Read the model definition and answer for the solid it produces. Units are mm, in the model's axes. A direction names the side the tool comes from. Give positions to 0.01 mm unless a question says otherwise; leave off trailing zeros. Order: outer loops, then holes, each group sorted by start corner. A loop starts at its lowest first (then second) coordinate and runs counter-clockwise, first axis right, second up.
```python
from build123d import *

# Parameters (mm, degrees)
SKETCH_1_W          = 25
SKETCH_1_H          = 8
EXTRUDE_1_DEPTH     = 5.5
SKETCH_3_W          = 7
SKETCH_3_H          = 1.5
EXTRUDE_3_DEPTH     = 9
SKETCH_4_W          = 5
SKETCH_4_H          = 1.5
EXTRUDE_4_DEPTH     = 3.5
SKETCH_5_R          = 1.25
CUT_EXTRUDE_1_DEPTH = 2


with BuildPart() as part:
    # 草图1 → 凸台-拉伸1 (new body)
    with BuildSketch(Plane(origin=(0, 0, 0), x_dir=(1, 0, 0), z_dir=(0, 1, 0))):
        Rectangle(SKETCH_1_W, SKETCH_1_H)
    extrude(amount=EXTRUDE_1_DEPTH)

    # 草图3 → 凸台-拉伸3 (add)
    with BuildSketch(Plane.XY.offset(4)):
        with Locations((-6, 2.75)):
            Rectangle(SKETCH_3_W, SKETCH_3_H)
        with Locations((6, 2.75)):
            Rectangle(SKETCH_3_W, SKETCH_3_H)
    extrude(amount=EXTRUDE_3_DEPTH)

    # 草图4 → 凸台-拉伸4 (add)
    with BuildSketch(Plane(origin=(0, 0, -4), x_dir=(-1, 0, 0), z_dir=(0, 0, -1))):
        with Locations((-6, 2.75)):
            Rectangle(SKETCH_4_W, SKETCH_4_H)
        with Locations((6, 2.75)):
            Rectangle(SKETCH_4_W, SKETCH_4_H)
    extrude(amount=EXTRUDE_4_DEPTH)

    # 草图5 → 切除-拉伸1 (cut)
    with BuildSketch(Plane(origin=(0, 5.5, 0), x_dir=(1, 0, 0), z_dir=(0, 1, 0))):
        with Locations(Location((-10.25, 0, 0), (0, 0, 270))):
            Circle(SKETCH_5_R)
        with Locations(Location((10.25, 0, 0), (0, 0, 90))):
            Circle(SKETCH_5_R)
    extrude(amount=-CUT_EXTRUDE_1_DEPTH, mode=Mode.SUBTRACT)


solid = part.part
```
1) Consider L1, parallel to X at y = 4.35, z = 0; L2, parallel to Z at x = 10.25, y = 4.5; L3, parallel to X at y = 2.6, z = 12.25. Determine where each line is inside the solid, lowest interval first.
Final values:
L1: x = -12.5 to -11.5, -9 to 9, 11.5 to 12.5
L2: z = -4 to -1.25, 1.25 to 4
L3: x = -9.5 to -2.5, 2.5 to 9.5
2) The part is cut by section C-C on x = -10.25. Determine the outline of the cut face in (y, z), and give its area (3 significant figures).
Final values:
outline: (0, -4) - (5.5, -4) - (5.5, -1.25) - (3.5, -1.25) - (3.5, 1.25) - (5.5, 1.25) - (5.5, 4) - (0, 4) - close
area: 39.0 mm2
3) Given pin 1 (1.6 mm diameter, centred on y = 3, z = -6, fed in from +X); pin 2 (2 mm diameter, centred on x = -9.5, y = 4, fed in from -Z); pin 3 (0.8 mm diameter, centred on y = 2.5, z = 9.5, fed in from +X), each flat-ended and moving along its own axis, determine where each tip first touches the part or whether it passes through.
Final values:
pin 1: stops at x = 8.5
pin 2: stops at z = -4
pin 3: stops at x = 9.5
4) The part is cut by section D-D on z = 0. Determine the outline of the cut face in (x, y).
Final values:
outline: (-12.5, 0) - (12.5, 0) - (12.5, 5.5) - (11.5, 5.5) - (11.5, 3.5) - (9, 3.5) - (9, 5.5) - (-9, 5.5) - (-9, 3.5) - (-11.5, 3.5) - (-11.5, 5.5) - (-12.5, 5.5) - close
5) The part is cut by section B-B on y = 4.2. Determine the outline of the cut face in (x, z), and give its area (3 significant figures).
Final values:
outline: (-12.5, -4) - (12.5, -4) - (12.5, 4) - (-12.5, 4) - close; hole circle Ø2.5 at (-10.25, 0); hole circle Ø2.5 at (10.25, 0)
area: 190 mm2
6) A tool of negligible diameter and unlimited length cuts with its end or side. For faces 1 (the face through (-6, 3.5, 8)), 2 (the face through (-3.5, 3, -6)), 3 (the face through (10, 3.5, 0)), 4 (the face through (6, 2, -6)), from which of +Z, -Z, +X, -X, +Y, -Y can it reach the whole face along a straight path? Write none if from no direction.
Final values:
face 1: +Z, +X, -X, +Y
face 2: -Z, +Y, -Y
face 3: +Y
face 4: -Z, +X, -X, -Y
7) For a pull along X with two mould halves and no side action, classify faces 5 (the face through (0, 5.5, 0)), 6 (the face through (3.5, 3, -6)), 7 (the face through (8.5, 3, -6)) as released by +X, released by -X, zero draft, split by the parting line, or undercut.
Final values:
face 5: zero draft
face 6: undercut
face 7: released by +X
8) The part is cut by section A-A on z = 5. Determine the outline of the cut face in (x, y).
Final values:
outline: (-9.5, 2) - (-2.5, 2) - (-2.5, 3.5) - (-9.5, 3.5) - close; (2.5, 2) - (9.5, 2) - (9.5, 3.5) - (2.5, 3.5) - close
